Check sheet for the modelled part. Datum: model origin and axes. Units: mm. Face numbers are marked on the shaded views. A direction names the side the tool comes from. Round coordinates to 2 decimals unless told otherwise and drop trailing zeros. Write each loop counter-clockwise with the first axis right and the second up, starting at its lowest first coordinate (ties: lowest second). Pieces come first, ordered by that corner, then holes. Notation, with made-up numbers: (15.25, 4) -> (74.25, 4) arc R21 ccw to (74.25, 42) -> close; hole circle Ø7 at (-34.5, 84). An arc over 180 degrees is marked (long way). One line per item, written item: value.
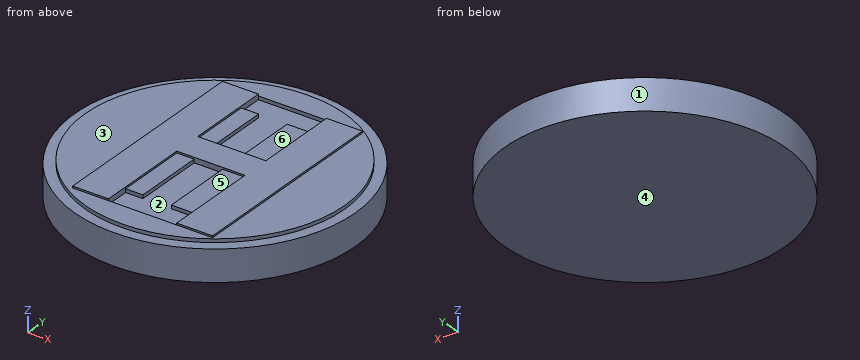
from build123d import *

# Parameters (mm, degrees)
SKETCH2_R                = 40
BOSS_EXTRUDE1_DEPTH      = 10
CUT_EXTRUDE1_START       = -1
CUT_EXTRUDE1_OUTLINE_R   = 40
CUT_EXTRUDE1_OUTLINE_R_2 = 37
CUT_EXTRUDE1_DEPTH       = 1
CUT_EXTRUDE1_2_DEPTH     = 0.5


# Read off the part's stored shape, not the designer's step: Cut-Extrude1
with BuildPart() as part:
    # Sketch2 → Boss-Extrude1 (new body)
    with BuildSketch(Plane.XY):
        Circle(SKETCH2_R)
    extrude(amount=-BOSS_EXTRUDE1_DEPTH)

    # Cut-Extrude1 outline → Cut-Extrude1 (cut)
    # profile 1 of 3: a face of its own
    with BuildSketch(Plane.XY.offset(CUT_EXTRUDE1_START)):
        Circle(CUT_EXTRUDE1_OUTLINE_R)
        Circle(CUT_EXTRUDE1_OUTLINE_R_2, mode=Mode.SUBTRACT)
    # profile 2 of 3: a face of its own
    with BuildSketch(Plane.XY.offset(CUT_EXTRUDE1_START)):
        Polygon((-9.007120253, -30), (10.454905063, -30), (10.454905063, -23.164556962), (4.070411392, -23.164556962), (4.070411392, -2.658227848), (-4.058544304, -2.658227848), (-4.058544304, -23.164556962), (-9.007120253, -23.164556962), align=None)
    # profile 3 of 3: a face of its own
    with BuildSketch(Plane.XY.offset(CUT_EXTRUDE1_START)):
        Polygon((-4.058544304, 5.696202532), (4.070411392, 5.696202532), (4.070411392, 23.164556962), (10.454905063, 23.164556962), (10.454905063, 30), (-9.007120253, 30), (-9.007120253, 23.164556962), (-4.058544304, 23.164556962), align=None)
    extrude(amount=CUT_EXTRUDE1_DEPTH, mode=Mode.SUBTRACT)

    # Cut-Extrude1 2 outline → Cut-Extrude1 2 (add)
    with BuildSketch(Plane.XY):
        Polygon((10.454905063, 30), (10.454905063, 5.696202532), (-9.007120253, 5.696202532), (-9.007120253, 30), (-19.26028481, 30), (-19.26028481, -30), (-9.007120253, -30), (-9.007120253, -2.658227848), (10.454905063, -2.658227848), (10.454905063, -30), (20.719936709, -30), (20.719936709, 30), align=None)
    extrude(amount=CUT_EXTRUDE1_2_DEPTH)


solid = part.part
Item 1: Sectioned sample at A-A on y = 0. Enter the section's corners in (x, z).
Answer:
outline: (-40, -10) -> (40, -10) -> (40, -1) -> (37, -1) -> (37, 0) -> (20.72, 0) -> (20.72, 0.5) -> (-19.26, 0.5) -> (-19.26, 0) -> (-37, 0) -> (-37, -1) -> (-40, -1) -> close
Item 2: Depth check by flat-ended pin: P1, Ø9.5, axis at x = -3, y = -9.5, coming from the +Z side; P2, Ø1.5, axis at x = 21, y = 14, coming from the +Z side; P3, Ø0.8, axis at x = 2.5, z = -0.5, coming from the -Y side; P4, Ø0.6, axis at x = -12.5, z = 0.5, coming from the -Y side. Enter the tip coordinate at first touch or a pass-through.
Answer:
P1: stops at z = 0
P2: stops at z = 0.5
P3: stops at y = -36.94
P4: stops at y = -30
Item 3: Sectioned sample at C-C on z = -8.75. Enter the section's corners in (x, y).
Answer:
outline: circle Ø80 at (0, 0)
Item 4: Mould release check, pull along Y, two halves, no side actions. Record for the marked faces 1, 2 and 3: pulls with the +Y half, pulls with the -Y half, needs draft (parallel to the pull), parting line crosses it, or undercut.
Answer:
face 1: parting line crosses it
face 2: undercut
face 3: needs draft
Item 5: Tool access check on the marked faces 4, 5 and 6. Record the directions out of +Z, -Z, +X, -X, +Y, -Y that give a thin tool (end or side, any length) a straight path to the whole face; none if there is none.
Answer:
face 4: -Z, +X, -X, +Y, -Y
face 5: +Z, -Y
face 6: +Z, +Y
Item 6: Sectioned sample at B-B on x = 0. Enter the section's corners in (y, z).
Answer:
outline: (-40, -10) -> (40, -10) -> (40, -1) -> (37, -1) -> (37, 0) -> (30, 0) -> (30, -1) -> (5.7, -1) -> (5.7, 0.5) -> (-2.66, 0.5) -> (-2.66, -1) -> (-30, -1) -> (-30, 0) -> (-37, 0) -> (-37, -1) -> (-40, -1) -> close
Item 7: Thickness scan on line 1 (Y direction, x = 5, z = 0.25); line 2 (Z direction, x = -24.5, y = 27.5); line 3 (Y direction, x = 0, z = -3.5). Record the ranges inside material, lowest first.
Answer:
line 1: y = -2.66 to 5.7
line 2: z = -10 to 0
line 3: y = -40 to 40
Item 8: Sectioned sample at D-D on y = 19. Enter the section's corners in (x, z).
Answer:
outline: (-35.2, -10) -> (35.2, -10) -> (35.2, -1) -> (31.75, -1) -> (31.75, 0) -> (20.72, 0) -> (20.72, 0.5) -> (10.45, 0.5) -> (10.45, 0) -> (4.07, 0) -> (4.07, -1) -> (-4.06, -1) -> (-4.06, 0) -> (-9.01, 0) -> (-9.01, 0.5) -> (-19.26, 0.5) -> (-19.26, 0) -> (-31.75, 0) -> (-31.75, -1) -> (-35.2, -1) -> close
